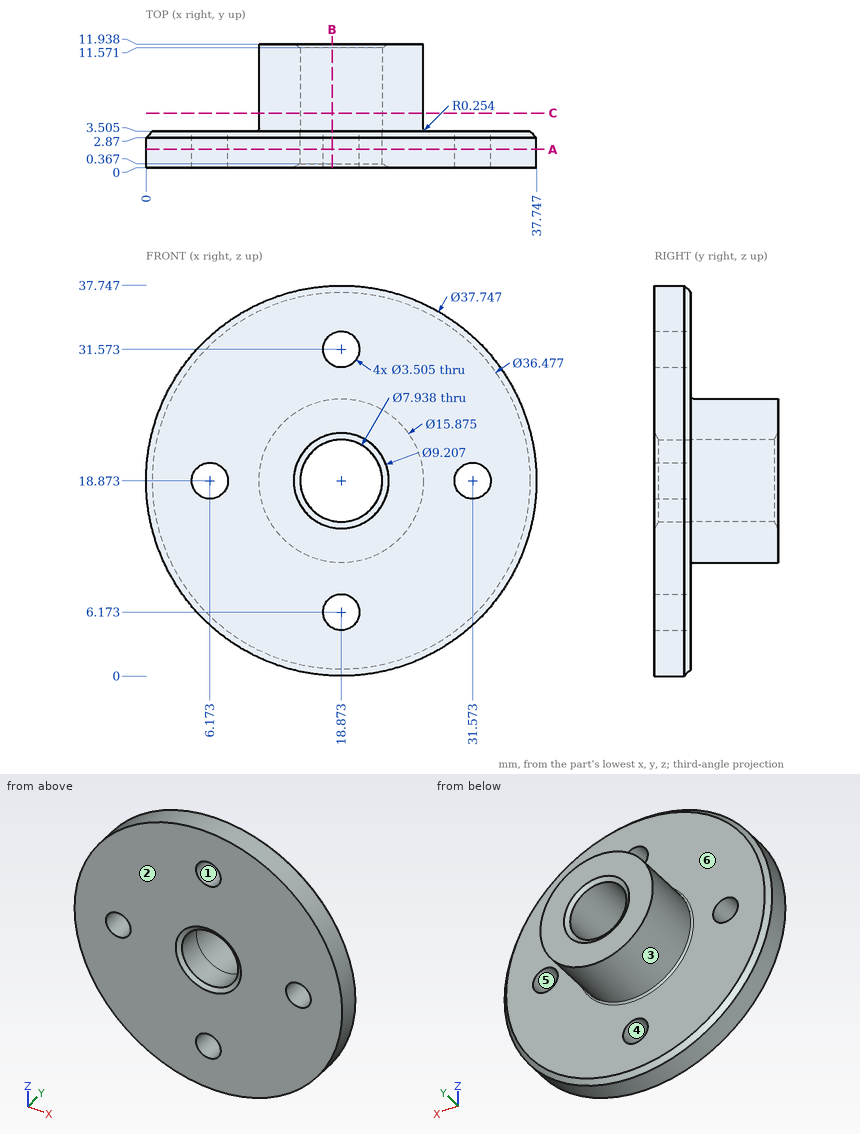
Design review of the part shown in the three views and the two pictorial views. Dimensions are in mm from the part's minimum x, y and z. A direction names the side the tool comes from. Give positions to 0.01 mm unless a question says otherwise; leave off trailing zeros. Loops run counter-clockwise (first coordinate to the right, second up) from the corner with the lowest first, then second, coordinate; pieces in that order, holes last. Notation, with made-up numbers: M -12.75,75 L 19.25,75 A23 cw 19.25,101 Z; hole C -15.5,1.25 d7. An arc over 180 degrees is marked long. Answer as a JSON object with one key per item and string values.
Item 1: Wall thickness on line 1 along X through (y, z) = (5.75, 19); line 2 along Y through (x, z) = (28, 31) (1 decimal); line 3 along X through (y, z) = (4.5, 16) (1 decimal): over which ranges is each line inside the solid? List them lowest first.
Output values:
{"line 1": "x = 10.94 to 14.91, 22.84 to 26.81", "line 2": "y = 0 to 3.5", "line 3": "x = 11.5 to 16.1, 21.6 to 26.3"}
Item 2: We need section C-C (y = 5.25). State the section outline as (x, z) points (1 decimal).
Output values:
{"outline": "C 18.9,18.9 d15.9; hole C 18.9,18.9 d7.9"}
Item 3: For P1, Ø4, axis at x = 31.57, z = 18.87, coming from the +Y side (1 decimal); P2, Ø10, axis at x = 27.5, z = 26.5, coming from the +Y side; P3, Ø1.5, axis at x = 11, y = 9, coming from the -Z side (1 decimal); P4, Ø5, axis at x = 10, y = 7.5, coming from the -Z side, all flat-tipped, find the tip position at first contact; note any pin that passes through.
Output values:
{"P1": "stops at y = 3.5", "P2": "stops at y = 11.94", "P3": "stops at z = 15.4", "P4": "stops at z = 14.14"}
Item 4: We need section A-A (y = 1.75). State the section outline as (x, z) points (1 decimal), and give its area (3 significant figures).
Output values:
{"outline": "C 18.9,18.9 d37.7; hole C 6.2,18.9 d3.5; hole C 18.9,18.9 d7.9; hole C 18.9,6.2 d3.5; hole C 18.9,31.6 d3.5; hole C 31.6,18.9 d3.5", "area": "1,030 mm2"}
Item 5: Mouldability with a two-part tool opening along Z and no side actions: class the marked faces 1, 2, 3 and 4 as pulls with the +Z half, pulls with the -Z half, needs draft (parallel to the pull), parting line crosses it, or undercut.
Output values:
{"face 1": "undercut", "face 2": "needs draft", "face 3": "parting line crosses it", "face 4": "undercut"}
Item 6: Machinability: for the marked faces 5 and 6, which of the approach directions +Z, -Z, +X, -X, +Y, -Y give a long, thin tool a straight path to every point of the face, cutting with its end or side? Answer none if there is none.
Output values:
{"face 5": "+Y, -Y", "face 6": "+Y"}
Item 7: We need section B-B (x = 18). Count the separate pieces of the cut face and the enclosed holes in it, and give its area (3 significant figures).
Output values:
{"separate pieces": "4", "enclosed holes": "0", "area": "151 mm2"}
